Verification items for the finished model (mm, model axes). Give positions to 0.01 mm unless a question says otherwise; leave off trailing zeros. Loops run counter-clockwise (first coordinate to the right, second up) from the corner with the lowest first, then second, coordinate; pieces in that order, holes last. Notation, with made-up numbers: M 15,-5 L 51,-5 A22 cw 51,11 Z; hole C 27.25,-7.75 d2. An arc over 180 degrees is marked long. Use CSV: the item, a comma, the result in double quotes.
Autodesk Inventor part; units mm, degrees
ref_plane "YZ Plane" through (0, 0, 0) normal (1, 0, 0) x (0, 1, 0)
ref_plane "XZ Plane" through (0, 0, 0) normal (0, 1, 0) x (-1, 0, 0)
ref_plane "XY Plane" through (0, 0, 0) normal (0, 0, 1) x (1, 0, 0)
sketch "Sketch1" plane through (0, 0, 0) normal (0, 1, 0) x (-1, 0, 0)
  line L0 (13.9277, -13.494) -> (-26.0723, -13.494)
  line L1 (-26.0723, -13.494) -> (-26.0723, 12.506)
  line L2 (-26.0723, 12.506) -> (13.9277, 12.506)
  line L3 (13.9277, 12.506) -> (13.9277, -13.494)
  point P0 (0, 0)
  dimension "d0" = 40
  dimension "d1" = 26
extrude "Extrusion1" add sketch "Sketch1" along normal blind 1
sketch "Sketch2" plane through (0, 0, 0) normal (0, -1, 0) x (1, 0, 0)
  circle A0 centre (24.0723, -11.494) radius 1
  line L0 (26.0723, -13.494) -> (-13.9277, -13.494)
  line L1 (26.0723, 12.506) -> (26.0723, -13.494)
  point P0 (0, 0)
  dimension "d4" = 2
  dimension "d5" = 2
  dimension "d6" = 2
extrude "Extrusion2" add sketch "Sketch2" along normal blind 3
pattern_linear "Rectangular Pattern1" count 2 spacing 22 along (-1, 0, 0) count 2 spacing 22 along (0, 0, 1) of "Extrusion2"
sketch "Sketch3" plane through (0, 1, 0) normal (0, 1, 0) x (1, 0, 0)
  line L0 (26.0723, -12.506) -> (26.0723, 13.494)
  line L1 (26.0723, 8.494) -> (0.0723, 8.494)
  line L2 (0.0723, 8.494) -> (0.0723, -7.506)
  line L3 (0.0723, -7.506) -> (26.0723, -7.506)
  line L4 (26.0723, -7.506) -> (26.0723, 8.494)
  line L5 (26.0723, 13.494) -> (-13.9277, 13.494)
  line L6 (-13.9277, -12.506) -> (26.0723, -12.506)
  circle A0 centre (-7.2277, 6.794) radius 3.3
  circle A1 centre (-7.2277, -5.806) radius 3.3
  line L7 (-13.9277, 13.494) -> (-13.9277, -12.506)
  point P0 (0, 0)
  dimension "d15" = 26
  dimension "d16" = 5
  dimension "d17" = 5
  dimension "d18" = 6.6
  dimension "d19" = 6.6
  dimension "d24" = 6.7
  dimension "d25" = 6.7
  dimension "d26" = 6.7
  dimension "d27" = 6.7
extrude "Extrusion3" cut sketch "Sketch3" against normal through all contours L3 L2 L1 L0 | A0 | A1
equation "\"d19\" = d18"
equation "\"d25\" = d24"
equation "\"d26\" = d25"
equation "\"d27\" = d24"
properties part number "dust_cover"
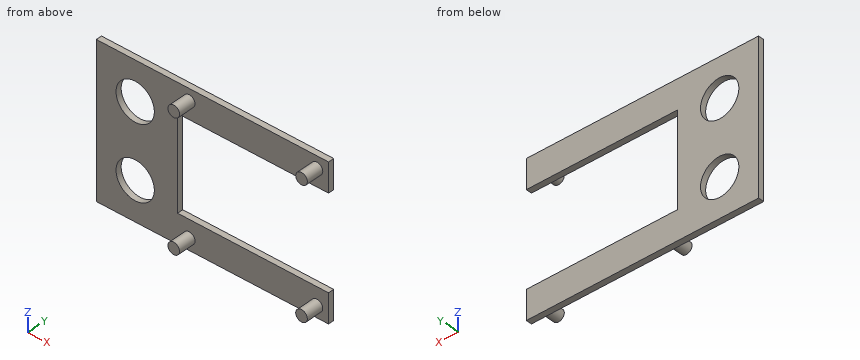
(1) Depth check by flat-ended pin: pin 1 Ø1.1 at (y, z) = (0.5, 2.5) entering from +X. Enter the tip coordinate at first touch or a pass-through.
Calculated:
pin 1,"stops at x = 0.07"
(2) Section check B-B on z = -9.5. Record the cut outline in (x, y), plus the area to 3 significant figures.
Calculated:
outline,"M -13.93,0 L -9.12,0 L -9.12,1 L -13.93,1 Z; M -5.34,0 L 26.07,0 L 26.07,1 L -5.34,1 Z"
area,"36.2 mm²"
(3) Scan lines: L1, parallel to Z at x = 0.5, y = 0.35; L2, parallel to Y at x = 0.5, z = -9; L3, parallel to X at y = 0.25, z = -7.25. Record each from-to range of solid material in increasing order. Write a range as from..to.
Calculated:
L1,"z = -13.49..-8.49, 7.51..12.51"
L2,"y = 0..1"
L3,"x = -13.93..-10.5, -3.96..0.07"
(4) Section check C-C on x = -10. Record the cut outline in (y, z).
Calculated:
outline,"M 0,-13.49 L 1,-13.49 L 1,-8.58 L 0,-8.58 Z; M 0,-5 L 1,-5 L 1,4.02 L 0,4.02 Z; M 0,7.6 L 1,7.6 L 1,12.51 L 0,12.51 Z"
(5) Section check D-D on y = 0.6. Record the cut outline in (x, z), plus the area to 3 significant figures.
Calculated:
outline,"M -13.93,-13.49 L 26.07,-13.49 L 26.07,-8.49 L 0.07,-8.49 L 0.07,7.51 L 26.07,7.51 L 26.07,12.51 L -13.93,12.51 Z; hole C -7.23,-6.79 d6.6; hole C -7.23,5.81 d6.6"
area,"556 mm²"
(6) Section check A-A on x = 18. Record the cut outline in (y, z), plus the area to 3 significant figures.
Calculated:
outline,"M 0,-13.49 L 1,-13.49 L 1,-8.49 L 0,-8.49 Z; M 0,7.51 L 1,7.51 L 1,12.51 L 0,12.51 Z"
area,"10.0 mm²"
